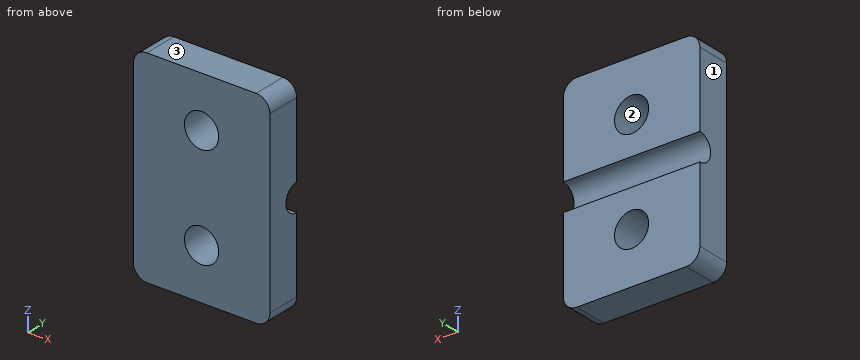
from build123d import *

# Parameters (mm, degrees)
EXTRUDE_1_DEPTH     = 10
SKETCH_2_R          = 1.25
CUT_EXTRUDE_1_DEPTH = 13.747548784
FILLET_1_R          = 1


with BuildPart() as part:
    # 草图1 → 凸台-拉伸1 (new body)
    with BuildSketch(Plane(origin=(0, 0, 0), x_dir=(0, 0, -1), z_dir=(1, 0, 0))):
        with BuildLine():
            Line((7.5, 1.25), (1, 1.25))
            ThreePointArc((1, 1.25), (0, 0.25), (-1, 1.25))
            Line((-1, 1.25), (-7.5, 1.25))
            Line((-7.5, 1.25), (-7.5, -1.25))
            Line((-7.5, -1.25), (7.5, -1.25))
            Line((7.5, -1.25), (7.5, 1.25))
        make_face()
    extrude(amount=EXTRUDE_1_DEPTH)

    # 草图2 → 切除-拉伸1 (cut, through all)
    with BuildSketch(Plane(origin=(0, 1.25, 0), x_dir=(1, 0, 0), z_dir=(0, 1, 0))):
        with Locations(Location((5, 3.75, 0), (0, 0, 270))):
            Circle(SKETCH_2_R)
        with Locations(Location((5, -3.75, 0), (0, 0, 270))):
            Circle(SKETCH_2_R)
    extrude(amount=-CUT_EXTRUDE_1_DEPTH, mode=Mode.SUBTRACT)

    # 圆角1
    fillet_1_edges = [part.edges().sort_by_distance(p)[0] for p in [
        (10, 0, 7.5),
        (10, 0, -7.5),
        (0, 0, -7.5),
        (0, 0, 7.5),
    ]]
    fillet(fillet_1_edges, radius=FILLET_1_R)


solid = part.part
Can you work these out from the model? Positions are in its coordinate system, mm. Face numbers are marked on the shaded views. Round coordinates to 2 decimals unless told otherwise and drop trailing zeros. Write each loop counter-clockwise with the first axis right and the second up, starting at its lowest first coordinate (ties: lowest second). Pieces come first, ordered by that corner, then holes. Notation, with made-up numbers: (-4.5, -15) -> (-0.5, -15) arc R7 cw to (-0.5, -2) -> close; hole circle Ø9 at (88.25, 13). An arc over 180 degrees is marked (long way). Use one line per item in the form item = value. Start each with the question number.
Q1. Imagine slicing it at B-B (z = 3). Please give me the cut outline in (x, y).
Q2. We'd pull the mould along Z, two halves only. Please class the marked faces 1, 2 and 3: +Z half, -Z half, draft (parallel to the pull), parting line (faces both ways), or undercut.
Q3. Imagine slicing it at A-A (x = 4). Please give me the cut outline in (y, z).
Q4. Imagine slicing it at D-D (y = 0.5). Please give me the cut outline in (x, z), then the cut area to 3 significant figures.
Q5. Imagine slicing it at C-C (y = -0.75). Please give me the cut outline in (x, z).
Q6. If I drill on probe 1 along X at (y, z) = (-0.25, 3.75); probe 2 along Z at (x, y) = (4.5, -1.05); probe 3 along Z at (x, y) = (4.75, 0.45), over which ranges is the centre line in solid material (lowest first)? Write a range as [from, to].
Q7. I'm going to push a flat-ended pin straight in: P1, Ø4, axis at x = 5, z = -3.75, coming from the -Y side. Where does the tip first touch, or does it pass through?
Worked out:
q1.outline = (0, -1.25) -> (4, -1.25) -> (4, 1.25) -> (0, 1.25) -> close; (6, -1.25) -> (10, -1.25) -> (10, 1.25) -> (6, 1.25) -> close
q2.face_1 = draft
q2.face_2 = undercut
q2.face_3 = +Z half
q3.outline = (-1.25, -7.5) -> (1.25, -7.5) -> (1.25, -4.5) -> (-1.25, -4.5) -> close; (-1.25, -3) -> (1.25, -3) -> (1.25, -1) arc R1 cw to (1.25, 1) -> (1.25, 3) -> (-1.25, 3) -> close; (-1.25, 4.5) -> (1.25, 4.5) -> (1.25, 7.5) -> (-1.25, 7.5) -> close
q4.outline = (0, -6.5) arc R1 ccw to (1, -7.5) -> (9, -7.5) arc R1 ccw to (10, -6.5) -> (10, -0.66) -> (0, -0.66) -> close; (0, 0.66) -> (10, 0.66) -> (10, 6.5) arc R1 ccw to (9, 7.5) -> (1, 7.5) arc R1 ccw to (0, 6.5) -> close; hole circle Ø2.5 at (5, -3.75); hole circle Ø2.5 at (5, 3.75)
q4.area = 126 mm^2
q5.outline = (0, -6.5) arc R1 ccw to (1, -7.5) -> (9, -7.5) arc R1 ccw to (10, -6.5) -> (10, 6.5) arc R1 ccw to (9, 7.5) -> (1, 7.5) arc R1 ccw to (0, 6.5) -> close; hole circle Ø2.5 at (5, -3.75); hole circle Ø2.5 at (5, 3.75)
q6.probe_1 = [0, 3.75], [6.25, 10]
q6.probe_2 = [-7.5, -4.9], [-2.6, 2.6], [4.9, 7.5]
q6.probe_3 = [-7.5, -4.97], [-2.53, -0.6], [0.6, 2.53], [4.97, 7.5]
q7.P1 = -1.25
